from build123d import *

# Parameters (mm, degrees)
F0_W        = 63
F0_H        = 43.5
F1_DEPTH    = 2
F2_R        = 5
F3_W        = 27.6
F3_H        = 5
F4_DEPTH    = 2
F5_R        = 2
F6_DEPTH    = 5
F7_W        = 45.5
F7_H        = 1.3
F8_DEPTH    = 1.7
F9_T1_DEPTH = 46.6629509039


# Not quite as in the source:
# - a fillet or chamfer that OpenCascade refuses, or shapes differently, is made with other operations: its cross-section is extruded or revolved along the edge and cut away or added


with BuildPart() as f1:
    # F0 (on Top) → F1 (new body)
    with BuildSketch(Plane.XY):
        with Locations((23.961127311, -16.9047259986)):
            Rectangle(F0_W, F0_H)
    extrude(amount=F1_DEPTH)

    # F2
    f2_edges = [f1.edges().sort_by_distance(p)[0] for p in [
        (-7.538873, 4.845274, 1),
        (55.461127, 4.845274, 1),
    ]]
    fillet(f2_edges, radius=F2_R)

    # F3 (on face) → F4 (join)
    with BuildSketch(Plane.XY.offset(2)):
        with Locations((23.961127311, 7.3452740014)):
            Rectangle(F3_W, F3_H)
        Polygon((10.161127311, -0.1547259986), (23.961127311, -0.1547259986), (37.761127311, -0.1547259986), (37.761127311, 4.8452740014), (10.161127311, 4.8452740014), align=None)
    extrude(amount=F4_DEPTH)

    # F5
    f5_edges = [f1.edges().sort_by_distance(p)[0] for p in [
        (10.161127, 9.845274, 3),
        (37.761127, 9.845274, 3),
    ]]
    fillet(f5_edges, radius=F5_R)

    # F3 (on face) → F6 (join)
    with BuildSketch(Plane.XY.offset(2)):
        Polygon((1.211127311, -37.2547259986), (1.211127311, -38.6547259986), (23.961127311, -38.6547259986), (46.711127311, -38.6547259986), (46.711127311, -37.2547259986), align=None)
    extrude(amount=F6_DEPTH)

    # F7 (on face) → F8 (join)
    with BuildSketch(Plane(origin=(0, -37.2547259986, 0), x_dir=(-1, 0, 0), z_dir=(0, 1, 0))):
        with Locations((-23.961127311, 6.35)):
            Rectangle(F7_W, F7_H)
    extrude(amount=F8_DEPTH)

    # F9: fillet of radius 8.9325901808 on 2 edges, made by hand

    # F9_s2 → F9_t1 (cut)
    with BuildSketch(Plane.XY.offset(-22.331475452)):
        with BuildLine():
            add(Edge.make_bspline(
                [(46.5285371302, -38.6547259986), (55.461127311, -38.6547259986), (55.461127311, -29.7221358179)],
                knots=[0, 0, 0, 1, 1, 1], degree=2, weights=[1, 1.5, 1]))
            Line((55.461127311, -29.7221358179), (55.461127311, -38.6547259986))
            Line((55.461127311, -38.6547259986), (46.5285371302, -38.6547259986))
        make_face()
        with BuildLine():
            add(Edge.make_bspline(
                [(-7.538872689, -29.7221358179), (-7.538872689, -38.6547259986), (1.3937174918, -38.6547259986)],
                knots=[0, 0, 0, 1, 1, 1], degree=2, weights=[1, 1.5, 1]))
            Line((1.3937174918, -38.6547259986), (-7.538872689, -38.6547259986))
            Line((-7.538872689, -38.6547259986), (-7.538872689, -29.7221358179))
        make_face()
    extrude(amount=F9_T1_DEPTH, mode=Mode.SUBTRACT)


solid = f1.part
CAD build for the part. Positions are in the model's coordinates, mm. A direction names the side the tool comes from. Give positions to 0.01 mm unless a question says otherwise; leave off trailing zeros. Loops run counter-clockwise (first coordinate to the right, second up) from the corner with the lowest first, then second, coordinate; pieces in that order, holes last. Notation, with made-up numbers: M 56,-16.75 L 69,-16.75 A20 cw 69,9.25 Z; hole C 33.25,-34 d2. An arc over 180 degrees is marked long. Answer in a Markdown table with one row per item. Add a question column.
Item 1: Band-saw the part on C-C on x = 5.5. Give the cut face in (y, z).
Item 2: Band-saw the part on A-A on x = 21. Give the cut face in (y, z).
Item 3: Drop flat-ended pins along their axis: P1, Ø1.5, axis at y = -37.5, z = 5, coming from the -X side; P2, Ø1.5, axis at x = 39.5, z = 4, coming from the +Y side; P3, Ø6, axis at x = 8.5, y = -18, coming from the +Z side. Give the stop position or say it passes through.
Item 4: Band-saw the part on B-B on y = -24.5. Give the cut face in (x, z), then the cut area to 3 significant figures.
Item 5: Tool access for faces 1 (the face through (1.211, -38, 5)), 2 (the face through (37.761, 4, 3)), 3 (the face through (24, -35.555, 6)), 4 (the face through (10.161, 4, 3)): list every direction of +Z, -Z, +X, -X, +Y, -Y with a clear straight run to the whole face (end or side of a thin tool).
Item 6: Mould opens along Z. For faces 5 (the face through (24, -37.255, 4)), 6 (the face through (24, 5, 4)), 7 (the face through (-7.539, -15, 1)) say: +Z half, -Z half, draft (parallel to the pull), parting line (faces both ways), or undercut.
Item 7: Band-saw the part on D-D on y = 2. Give the cut face in (x, z).
Item 8: Probe probe 1 along Y at (x, z) = (34.5, 3); probe 2 along Z at (x, y) = (39, -15); probe 3 along Z at (x, y) = (24.5, 7.5). List the from-to ranges inside material, lowest first.
Reply:
| question | item | result |
|---|---|---|
| 1 | outline | M -38.65,0 L 4.85,0 L 4.85,2 L -37.25,2 L -37.25,5.7 L -35.55,5.7 L -35.55,7 L -38.65,7 Z |
| 2 | outline | M -38.65,0 L 4.85,0 L 4.85,2 L 9.85,2 L 9.85,4 L -0.15,4 L -0.15,2 L -37.25,2 L -37.25,5.7 L -35.55,5.7 L -35.55,7 L -38.65,7 Z |
| 3 | P1 | stops at x = 1.21 |
| 3 | P2 | stops at y = -37.25 |
| 3 | P3 | stops at z = 2 |
| 4 | outline | M -7.54,0 L 55.46,0 L 55.46,2 L -7.54,2 Z |
| 4 | area | 126 mm^2 |
| 5 | face 1 | +Z, -X, +Y, -Y |
| 5 | face 2 | +Z, +X, +Y |
| 5 | face 3 | +Z, +X, -X, +Y |
| 5 | face 4 | +Z, -X, +Y |
| 6 | face 5 | undercut |
| 6 | face 6 | +Z half |
| 6 | face 7 | draft |
| 7 | outline | M -7.05,0 L 54.97,0 L 54.97,2 L 37.76,2 L 37.76,4 L 10.16,4 L 10.16,2 L -7.05,2 Z |
| 8 | probe 1 | y = -38.65 to -37.25, -0.15 to 9.85 |
| 8 | probe 2 | z = 0 to 2 |
| 8 | probe 3 | z = 2 to 4 |
